from build123d import *

# Parameters (mm, degrees)
F1_DEPTH  = 32
F3_DEPTH  = 19
F5_DEPTH  = 11
F6_R      = 10
F7_DEPTH  = 25
F8_R      = 19.5
F9_DEPTH  = 12
F11_R     = 7.5
F12_DEPTH = 70
F14_DEPTH = 32


with BuildPart() as f1:
    # F0 (on Right) → F1 (new body, symmetric)
    with BuildSketch(Plane.YZ):
        with BuildLine():
            Line((-45, 77.9422863406), (0, 0))
            Line((0, 0), (140, 0))
            Line((140, 0), (140, 19))
            Line((140, 19), (16.7431578065, 19))
            ThreePointArc((16.7431578065, 19), (11.7431578065, 20.3397459622), (8.0829037687, 24))
            Line((8.0829037687, 24), (-19.0455173281, 70.9878036687))
            Line((-19.0455173281, 70.9878036687), (36.3801085141, 102.9878036687))
            Line((36.3801085141, 102.9878036687), (26.8801085141, 119.4422863406))
            Line((26.8801085141, 119.4422863406), (-45, 77.9422863406))
        make_face()
    extrude(amount=F1_DEPTH, both=True)

    # F2 (on face) → F3 (cut, through all)
    with BuildSketch(Plane(origin=(0, -45, 77.9422863406), x_dir=(1, 0, 0), z_dir=(0, -0.5, 0.8660254038))):
        with BuildLine():
            Line((32, 83), (0, 83))
            ThreePointArc((0, 83), (22.627416998, 73.627416998), (32, 51))
            Line((32, 51), (32, 83))
        make_face()
        with BuildLine():
            Line((-32, 83), (-32, 51))
            ThreePointArc((-32, 51), (-22.627416998, 73.627416998), (0, 83))
            Line((0, 83), (-32, 83))
        make_face()
        Polygon((-106.2661910977, 51), (-32, 51), (-32, 83), (0, 83), (32, 83), (32, 51), (106.2661910977, 51), (106.2661910977, 125.2661910977), (-106.2661910977, 125.2661910977), align=None)
    extrude(amount=-F3_DEPTH, mode=Mode.SUBTRACT)

    # F4 (on Right) → F5 (cut, symmetric)
    with BuildSketch(Plane.YZ):
        Polygon((-36.8038475773, 75.7461339179), (80.5091410398, 143.4768194754), (54.8271117013, 187.9593991312), (-109.3994230032, 93.1431651115), (-58.7173936647, 5.3593152665), (-11.8038475773, 32.4448637287), align=None)
    extrude(amount=F5_DEPTH, both=True, mode=Mode.SUBTRACT)

    # F6 (on face) → F7 (cut, symmetric)
    with BuildSketch(Plane(origin=(0, -42, 72.7461339179), x_dir=(1, 0, 0), z_dir=(0, -0.5, 0.8660254038))):
        with Locations((0, 51)):
            Circle(F6_R)
    extrude(amount=F7_DEPTH, both=True, mode=Mode.SUBTRACT)

    # F8 (on face) → F9 (cut)
    with BuildSketch(Plane(origin=(0, -45, 77.9422863406), x_dir=(1, 0, 0), z_dir=(0, -0.5, 0.8660254038))):
        with Locations((0, 51)):
            Circle(F8_R)
    extrude(amount=-F9_DEPTH, mode=Mode.SUBTRACT)

    # F11 (on offset) → F12 (join)
    with BuildSketch(Plane(origin=(0, 125, 0), x_dir=(-1, 0, 0), z_dir=(0, 1, 0))):
        with BuildLine():
            Line((-12.5, 44), (-12.5, 19))
            Line((-12.5, 19), (12.5, 19))
            Line((12.5, 19), (12.5, 44))
            ThreePointArc((12.5, 44), (0, 56.5), (-12.5, 44))
        make_face()
        with Locations((0, 44)):
            Circle(F11_R, mode=Mode.SUBTRACT)
    extrude(amount=-F12_DEPTH)

    # F13 (on Right) → F14 (cut, symmetric)
    with BuildSketch(Plane.YZ):
        Polygon((110, 97.3418423458), (70, 97.3418423458), (70, 26), (90, 26), (110, 26), align=None)
    extrude(amount=F14_DEPTH, both=True, mode=Mode.SUBTRACT)


solid = f1.part
Could you check a few things on this model? Use its own coordinates, in mm. A direction names the side the tool comes from. Give positions to 0.01 mm unless a question says otherwise; leave off trailing zeros. Order: outer loops, then holes, each group sorted by start corner. A loop starts at its lowest first (then second) coordinate and runs counter-clockwise, first axis right, second up.
1. Suppose I cut it at B-B (x = -23.5). Write out the boundary of the cut face in (y, z), plus the area to 3 significant figures.
Answers below:
outline: (-45, 77.94) - (0, 0) - (140, 0) - (140, 19) - (16.74, 19) arc R10 cw to (8.08, 24) - (-19.05, 70.99) - (27.48, 97.85) - (17.98, 114.3) - close
area: 5,190 mm2
2. I need wall thicknesses on L1, parallel to Z at x = 0, y = 117.5; L2, parallel to Z at x = -22.5, y = 112; L3, parallel to Y at x = 10, z = 48. Which ranges of each line are inside material? Lowest first, please.
Answers below:
L1: z = 0 to 36.5, 51.5 to 56.5
L2: z = 0 to 19
L3: y = -20.78 to -5.77, 55 to 70, 110 to 125
3. Suppose I cut it at C-C (y = 128.5). Write out the boundary of the cut face in (x, z), plus the area to 3 significant figures.
Answers below:
outline: (-32, 0) - (32, 0) - (32, 19) - (-32, 19) - close
area: 1,220 mm2
4. Thinking about a two-plate mould opening in Z: for faces 1 (the flat face through (0.15, 24.43, 111.1)), 2 (the flat face through (0, 69, 0)), 3 (the flat face through (0.154, -24.129, 53.792)), which applies, +Z half, -Z half, draft (parallel to the pull), parting line (faces both ways), or undercut?
Answers below:
face 1: +Z half
face 2: -Z half
face 3: undercut
5. Suppose I cut it at D-D (x = 28.5). Write out the boundary of the cut face in (y, z).
Answers below:
outline: (-45, 77.94) - (0, 0) - (140, 0) - (140, 19) - (16.74, 19) arc R10 cw to (8.08, 24) - (-19.05, 70.99) - (21.27, 94.26) - (11.77, 110.72) - close
6. For pin 1 (20 mm diameter, centred on x = 0.5, z = 39, fed in from -Y); pin 2 (13.5 mm diameter, centred on y = 19.5, z = 113, fed in from +X); pin 3 (13.5 mm diameter, centred on y = 20, z = 112.5, fed in from -X); pin 4 (6 mm diameter, centred on x = -13.5, y = 2, fed in from -Z), each with a flat end and sliding along its axis, tell me the tip position at first contact or that it passes through.
Answers below:
pin 1: stops at y = -21.36
pin 2: stops at x = 27.92
pin 3: stops at x = -27.82
pin 4: stops at z = 0
7. Which directions (+Z, -Z, +X, -X, +Y, -Y) give clear straight access to the entire face, cutting with the end or side of a thin tool? Please do faces 4 (the flat face through (0, 70, 35)), 5 (the flat face through (11, 21, 112)), 6 (the flat face through (0.45, -5.29, 47.16)).
Answers below:
face 4: +Z, +X, -X
face 5: +Z, -Y
face 6: +X, -X
8. Suppose I cut it at A-A (y = 82). Write out the boundary of the cut face in (x, z).
Answers below:
outline: (-32, 0) - (32, 0) - (32, 19) - (12.5, 19) - (12.5, 26) - (-12.5, 26) - (-12.5, 19) - (-32, 19) - close
